Source: CAD feature listing. Evaluate the final solid. Frame: model axes, mm. Give positions to 0.01 mm unless a question says otherwise; leave off trailing zeros. Order: outer loops, then holes, each group sorted by start corner. A loop starts at its lowest first (then second) coordinate and runs counter-clockwise, first axis right, second up. Notation, with made-up numbers: M 34,4.5 L 83,4.5 A29 cw 83,25.5 Z; hole C 71.25,22 d8. An arc over 180 degrees is marked long. One line per question, with ' | ' between items. Start each with the question number.
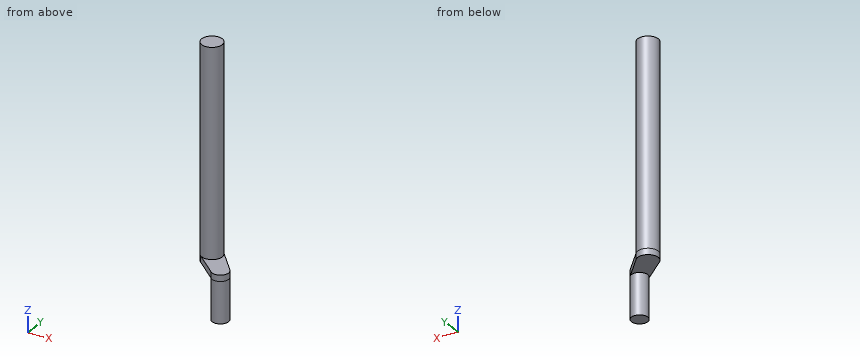
from build123d import *

# Parameters (mm, degrees)
SKETCH1_R           = 10
BOSS_EXTRUDE1_DEPTH = 200
BOSS_EXTRUDE2_DEPTH = 6
SKETCH4_R           = 8
BOSS_EXTRUDE3_DEPTH = 40


with BuildPart() as part:
    # Sketch1 → Boss-Extrude1 (new body)
    with BuildSketch(Plane.XY):
        Circle(SKETCH1_R)
    extrude(amount=BOSS_EXTRUDE1_DEPTH)

    # Sketch2 → Boss-Extrude2 (add)
    with BuildSketch(Plane(origin=(0, 0, 0), x_dir=(-1, 0, 0), z_dir=(0, 0, -1))):
        with BuildLine():
            Line((-27.117555988, -16.267702887), (-7.592066465, 6.508496508))
            ThreePointArc((-7.592066465, 6.508496508), (6.999097965, 7.142312488), (6.660920323, -7.458695627))
            Line((6.660920323, -7.458695627), (-15.715166558, -27.441456595))
            ThreePointArc((-15.715166558, -27.441456595), (-26.643181188, -27.188350084), (-27.117555988, -16.267702887))
        make_face()
    extrude(amount=BOSS_EXTRUDE2_DEPTH)

    # Sketch4 → Boss-Extrude3 (add)
    with BuildSketch(Plane(origin=(0, 0, -6), x_dir=(-1, 0, 0), z_dir=(0, 0, -1))):
        with Locations((-21.043902817, -21.474500093)):
            Circle(SKETCH4_R)
    extrude(amount=BOSS_EXTRUDE3_DEPTH)


solid = part.part
Item 1: Pin query (flat end, axial travel): pin 1 Ø11 at (x, y) = (5.5, -6.5) entering from -Z; pin 2 Ø2 at (x, z) = (22.5, -16) entering from -Y; pin 3 Ø10 at (x, y) = (24.5, -24.5) entering from +Z. Return the tip coordinate at first contact, or that it passes through.
Item 2: Line query: line 1 (Z direction, x = 2.5, y = -13.5); line 2 (X direction, y = 1, z = 178); line 3 (Z direction, x = -1, y = 4). Output: solid intervals per line, ascending.
Item 3: Cut plane B-B on z = 162.5. Return the cut outline in (x, y), and give its area (3 significant figures).
Item 4: Cut plane D-D on y = 0. Return the cut outline in (x, z).
Item 5: Cut plane A-A on y = -19. Return the cut outline in (x, z), and give its area (3 significant figures).
Item 6: Cut plane C-C on x = 0. Return the cut outline in (y, z).
Results are:
1) pin 1: stops at z = -6 | pin 2: stops at y = -29.46 | pin 3: stops at z = 0
2) line 1: z = -6 to 0 | line 2: x = -9.95 to 9.95 | line 3: z = -6 to 200
3) outline: C 0,0 d20 | area: 314 mm2
4) outline: M -10,-6 L 13.17,-6 L 13.17,0 L 10,0 L 10,200 L -10,200 Z
5) outline: M 6.26,-6 L 13.44,-6 L 13.44,-46 L 28.65,-46 L 28.65,0 L 6.26,0 Z | area: 743 mm2
6) outline: M -13.41,-6 L 10,-6 L 10,200 L -10,200 L -10,0 L -13.41,0 Z
